from build123d import *

# Parameters (mm, degrees)
SKETCH1_W           = 179.900000372
SKETCH1_H           = 203.2
SKETCH1_R           = 3.175
BOSS_EXTRUDE1_DEPTH = 3.175
FILLET1_R           = 6.35


with BuildPart() as part:
    # Sketch1 → Boss-Extrude1 (new body)
    with BuildSketch(Plane(origin=(0, 0, 0), x_dir=(1, 0, 0), z_dir=(0, 1, 0))):
        with Locations((57.15, 101.6)):
            Rectangle(SKETCH1_W, SKETCH1_H)
        with Locations((-26.450000186, 6.35)):
            Circle(SKETCH1_R, mode=Mode.SUBTRACT)
        with Locations((140.750000186, 6.35)):
            Circle(SKETCH1_R, mode=Mode.SUBTRACT)
        with Locations((-26.450000186, 196.85)):
            Circle(SKETCH1_R, mode=Mode.SUBTRACT)
        with Locations((140.750000186, 196.85)):
            Circle(SKETCH1_R, mode=Mode.SUBTRACT)
    extrude(amount=BOSS_EXTRUDE1_DEPTH)

    # Fillet1
    fillet1_edges = [part.edges().sort_by_distance(p)[0] for p in [
        (-32.800000186, 1.5875, -203.2),
        (147.100000186, 1.5875, -203.2),
        (147.100000186, 1.5875, 0),
        (-32.800000186, 1.5875, 0),
    ]]
    fillet(fillet1_edges, radius=FILLET1_R)


solid = part.part
Work out the finished part from the listing and answer in its coordinate system (mm). Give positions to 0.01 mm unless a question says otherwise; leave off trailing zeros.
Q1. For a pull along Z with two mould halves and no side action, classify faces 1 (the face through (56, 3.175, -103)), 2 (the face through (-30.99, 1.61, -201.29)), 3 (the face through (140.06, 1.57, -193.75)) as released by +Z, released by -Z, zero draft, split by the parting line, or undercut.
Answer:
face 1: zero draft
face 2: released by -Z
face 3: undercut
Q2. Straight lines are drawn through the part: L1, parallel to Z at x = -26.45, y = 1.55 (3 decimals); L2, parallel to X at y = 0.8, z = -196.85 (3 decimals). For each, find the intervals that lie inside material, in ascending order.
Answer:
L1: z = -203.2 to -200.025, -193.675 to -9.525, -3.175 to 0
L2: x = -32.8 to -29.625, -23.275 to 137.575, 143.925 to 147.1
Q3. Given pin 1 (4 mm diameter, centred on x = 140.75, z = -196.85, fed in from -Y), flat-ended and moving along its own axis, determine where the tip first touches the part or whether it passes through.
Answer:
pin 1: passes through
